Answer from the drawing. Dimensions are ordinates in mm from the lowest x, y and z of the part. Give positions to 0.01 mm unless a question says otherwise; leave off trailing zeros. Loops run counter-clockwise (first coordinate to the right, second up) from the corner with the lowest first, then second, coordinate; pieces in that order, holes last. Notation, with made-up numbers: (38, 77.5) -> (94, 77.5) arc R16 cw to (94, 87.5) -> close; hole circle Ø11 at (-8, 72). An arc over 180 degrees is marked (long way). Write each question's results on one line, items separated by ' | '. Start each with the question number.
Item 1: Section A-A on x = 6.25 is taken. Write down the section's boundary in (y, z).
Item 2: Section B-B on y = 19.5 is taken. Write down the section's boundary in (x, z), and give its area (3 significant figures).
Item 3: Find the intervals of material crossed by line 1 (Y direction, x = 7.75, z = 8.5); line 2 (Z direction, x = 8.75, y = 13); line 3 (X direction, y = 12.25, z = 4), in increasing order.
Item 4: Each of these flat-tipped pins is pushed along its axis until it touches: P1, Ø3, axis at x = 8, z = 8.5, coming from the -Y side; P2, Ø5, axis at x = 4.5, z = 11.5, coming from the -Y side; P3, Ø5, axis at y = 6.5, z = 8.5, coming from the -X side. Where does it stop, or does it pass through?
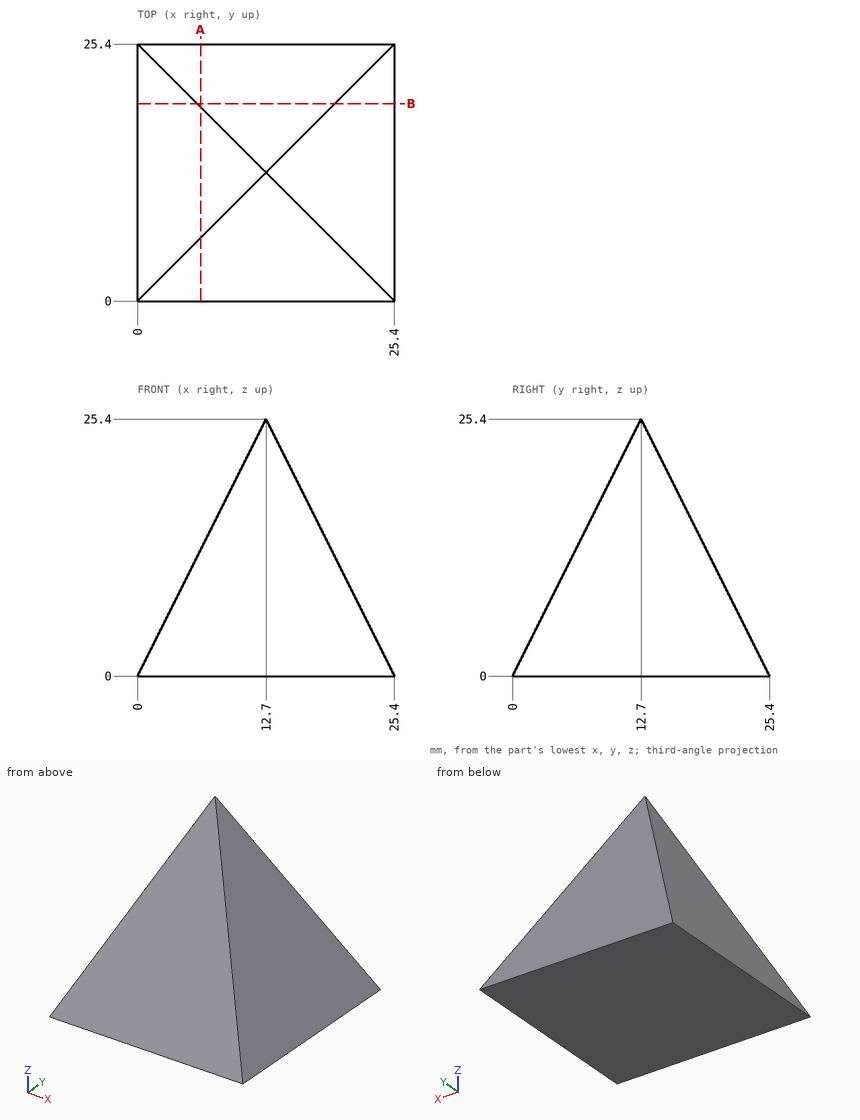
Findings:
1) outline: (0, 0) -> (25.4, 0) -> (19.15, 12.5) -> (6.25, 12.5) -> close
2) outline: (0, 0) -> (25.4, 0) -> (19.5, 11.8) -> (5.9, 11.8) -> close | area: 230 mm2
3) line 1: 4.25 to 21.15 | line 2: 0 to 17.5 | line 3: 2 to 23.4
4) P1: y = 3.5 | P2: y = 4.5 | P3: x = 3
